Could you check a few things on this model? Use its own coordinates, in mm. A direction names the side the tool comes from. Give positions to 0.01 mm unless a question says otherwise; leave off trailing zeros. Loops run counter-clockwise (first coordinate to the right, second up) from the corner with the lowest first, then second, coordinate; pieces in that order, holes last. Notation, with made-up numbers: (47.5, -10) -> (103.5, -10) arc R23 cw to (103.5, 21) -> close; hole circle Ø1 at (5, 10). An arc over 180 degrees is marked (long way). Write item = value, one per line. Start each with the question number.
1) I want a section at C-C (x = 1.25). List the corners of the cut face in (y, z) for me (3 decimals).
2) I'm going to push flat-ended pins straight in: pin 1 Ø10 at (x, y) = (-6.5, 0.5) entering from +Z; pin 2 Ø10 at (y, z) = (0.5, 19.5) entering from -X; pin 3 Ø2 at (x, y) = (3.5, 0.5) entering from +Z (3 decimals). Where does each tip first touch, or does it pass through?
3) If we mould it in two halves opening along Y, with no side actions, what happens to faces 4 (the face through (-9.462, 0, 4)), 5 (the face through (6.16, -4, 12)), 6 (the face through (0, -10.643, 12))? For each: +Y half, -Y half, draft (parallel to the pull), parting line (faces both ways), or undercut.
4) I want a section at B-B (y = 0.75). List the corners of the cut face in (x, z) for me (1 decimal), and give its area (3 significant figures).
5) I want a section at D-D (z = 17.75). List the corners of the cut face in (x, y) for me.
6) I want a section at A-A (z = 5). List the corners of the cut face in (x, y) for me, and give its area (3 significant figures).
7) On a 3-axis mill with a long thin cutter (end or side, diameter ignored), from which of +Z, -Z, +X, -X, +Y, -Y can I reach the whole of each face in a straight line? I mean faces 1 (the face through (-1.08, 0, 4)), 2 (the face through (7.049, 0, 21)), 3 (the face through (6, -0.356, 23)). Say none if no direction works.
8) I need wall thicknesses on probe 1 along Z at (x, y) = (6.25, 8.5) (3 decimals); probe 2 along Y at (x, z) = (3, 2.5); probe 3 along Y at (x, z) = (-7, 6.75). Which ranges of each line are inside material? Lowest first, please. Write a range as from..to.
from build123d import *

# Parameters (mm, degrees)
SKETCH1_W           = 18.923
SKETCH1_H           = 21.2852
BOSS_EXTRUDE1_DEPTH = 23.495
CUT_EXTRUDE1_DEPTH  = 18.1102
SKETCH3_W           = 6.223
SKETCH3_H           = 4.0132
CUT_EXTRUDE2_DEPTH  = 3.4798
SKETCH4_W           = 2.9718
SKETCH4_H           = 5.6642
CUT_EXTRUDE3_DEPTH  = 1.4478
SKETCH5_W           = 1.27
SKETCH5_H           = 17.4752
CUT_EXTRUDE4_DEPTH  = 16.51
SKETCH7_R           = 0.9525
CUT_EXTRUDE6_DEPTH  = 5.08


with BuildPart() as part:
    # Sketch1 → Boss-Extrude1 (new body)
    with BuildSketch(Plane.XY):
        Rectangle(SKETCH1_W, SKETCH1_H)
    extrude(amount=BOSS_EXTRUDE1_DEPTH)

    # Sketch2 → Cut-Extrude1 (cut)
    with BuildSketch(Plane.XY.offset(23.495)):
        Polygon((-9.4615, 6.8834), (-9.4615, -6.8834), (-1.0795, -6.8834), (-1.0795, -7.4676), (6.1595, -7.4676), (6.1595, -0.3556), (5.1435, -0.3556), (5.1435, 2.0066), (4.1275, 2.0066), (4.1275, 7.4676), (-1.0795, 7.4676), (-1.0795, 6.8834), align=None)
    extrude(amount=-CUT_EXTRUDE1_DEPTH, mode=Mode.SUBTRACT)

    # Sketch3 → Cut-Extrude2 (cut)
    with BuildSketch(Plane.XY.offset(5.3848)):
        with Locations((2.032, 0)):
            Rectangle(SKETCH3_W, SKETCH3_H)
    extrude(amount=-CUT_EXTRUDE2_DEPTH, mode=Mode.SUBTRACT)

    # Sketch4 → Cut-Extrude3 (cut)
    with BuildSketch(Plane.XY.offset(5.3848)):
        with Locations((4.6736, -4.6355)):
            Rectangle(SKETCH4_W, SKETCH4_H)
    extrude(amount=-CUT_EXTRUDE3_DEPTH, mode=Mode.SUBTRACT)

    # Sketch5 → Cut-Extrude4 (cut)
    with BuildSketch(Plane.ZY.offset(9.4615)):
        with Locations((20.955, 0)):
            Rectangle(SKETCH5_W, SKETCH5_H)
    extrude(amount=-CUT_EXTRUDE4_DEPTH, mode=Mode.SUBTRACT)

    # Sketch7 → Cut-Extrude6 (cut)
    with BuildSketch(Plane.XY.offset(23.495)):
        with Locations((5.3975, 6.1976)):
            Circle(SKETCH7_R)
    extrude(amount=-CUT_EXTRUDE6_DEPTH, mode=Mode.SUBTRACT)


solid = part.part
Answer list:
q1.outline = (-10.643, 0) -> (10.643, 0) -> (10.643, 23.495) -> (7.468, 23.495) -> (7.468, 21.59) -> (8.738, 21.59) -> (8.738, 20.32) -> (7.468, 20.32) -> (7.468, 5.385) -> (2.007, 5.385) -> (2.007, 1.905) -> (-2.007, 1.905) -> (-2.007, 5.385) -> (-7.468, 5.385) -> (-7.468, 20.32) -> (-8.738, 20.32) -> (-8.738, 21.59) -> (-7.468, 21.59) -> (-7.468, 23.495) -> (-10.643, 23.495) -> close
q2.pin_1 = 5.38
q2.pin_2 = 4.13
q2.pin_3 = 1.905
q3.face_4 = draft
q3.face_5 = undercut
q3.face_6 = -Y half
q4.outline = (-9.5, 0) -> (9.5, 0) -> (9.5, 23.5) -> (5.1, 23.5) -> (5.1, 21.6) -> (7, 21.6) -> (7, 20.3) -> (5.1, 20.3) -> (5.1, 1.9) -> (-1.1, 1.9) -> (-1.1, 5.4) -> (-9.5, 5.4) -> close
q4.area = 156 mm^2
q5.outline = (-9.46, -10.64) -> (9.46, -10.64) -> (9.46, 10.64) -> (-9.46, 10.64) -> (-9.46, 6.88) -> (-1.08, 6.88) -> (-1.08, 7.47) -> (4.13, 7.47) -> (4.13, 2.01) -> (5.14, 2.01) -> (5.14, -0.36) -> (6.16, -0.36) -> (6.16, -7.47) -> (-1.08, -7.47) -> (-1.08, -6.88) -> (-9.46, -6.88) -> close
q6.outline = (-9.46, -10.64) -> (9.46, -10.64) -> (9.46, 10.64) -> (-9.46, 10.64) -> close; hole (-1.08, -2.01) -> (3.19, -2.01) -> (3.19, -7.47) -> (6.16, -7.47) -> (6.16, -1.8) -> (5.14, -1.8) -> (5.14, 2.01) -> (-1.08, 2.01) -> close
q6.area = 361 mm^2
q7.face_1 = +Z
q7.face_2 = -X
q7.face_3 = +Z, -X
q8.probe_1 = 0..20.32, 21.59..23.495
q8.probe_2 = -10.64..-2.01, 2.01..10.64
q8.probe_3 = -10.64..-6.88, 6.88..10.64
